Autodesk Inventor part; units mm, degrees
ref_plane "YZ Plane" through (0, 0, 0) normal (1, 0, 0) x (0, 1, 0)
ref_plane "XZ Plane" through (0, 0, 0) normal (0, 1, 0) x (-1, 0, 0)
ref_plane "XY Plane" through (0, 0, 0) normal (0, 0, 1) x (1, 0, 0)
sketch "Sketch1" plane through (0, 0, 0) normal (0, 0, 1) x (1, 0, 0)
  line L0 (52.5, 53) -> (52.5, -53)
  line L1 (-52.5, 53) -> (52.5, 53)
  line L2 (52.5, 53) -> (-52.5, 53)
  line L3 (-52.5, 53) -> (-52.5, -53)
  line L4 (-52.5, -53) -> (52.5, -53)
  line L5 (52.5, -53) -> (52.5, 53)
  line L6 (50.5, -51) -> (50.5, 51)
  line L7 (50.5, 51) -> (-50.5, 51)
  line L8 (50.5, 51) -> (-50.5, 51)
  line L9 (-50.5, 51) -> (-50.5, -51)
  line L10 (-50.5, -51) -> (50.5, -51)
  line L11 (50.5, -51) -> (50.5, 51)
  point P0 (0, 0)
extrude "Extrusion1" add sketch "Sketch1" along normal blind 10
sketch "Sketch2" plane through (0, 0, 0) normal (0, 0, -1) x (-1, 0, 0)
  circle A0 centre (-46, 46.5) radius 1.5
  line L0 (-50.5, 51) -> (-50.5, 42)
  line L1 (-41.5, 51) -> (-50.5, 51)
  line L2 (-41.5, 51) -> (-41.5, 42)
  line L3 (-41.5, 42) -> (-50.5, 42)
  circle A1 centre (-46, -46.5) radius 1.5
  line L4 (-41.5, -42) -> (-41.5, -51)
  line L5 (-50.5, -51) -> (-41.5, -51)
  line L6 (-50.5, -42) -> (-50.5, -51)
  line L7 (-50.5, -42) -> (-41.5, -42)
  circle A2 centre (46, -46.5) radius 1.5
  line L8 (50.5, -51) -> (50.5, -42)
  line L9 (41.5, -51) -> (50.5, -51)
  line L10 (41.5, -51) -> (41.5, -42)
  line L11 (41.5, -42) -> (50.5, -42)
  circle A3 centre (46, 46.5) radius 1.5
  line L12 (41.5, 42) -> (41.5, 51)
  line L13 (50.5, 51) -> (41.5, 51)
  line L14 (50.5, 42) -> (50.5, 51)
  line L15 (50.5, 42) -> (41.5, 42)
  point P0 (0, 0)
extrude "Extrusion2" add sketch "Sketch2" against normal blind 10
sketch "Sketch3" plane through (0, 0, 10) normal (0, 0, 1) x (1, 0, 0)
  line L0 (43.467, -7.68) -> (39.533, -7.68)
  line L1 (39.533, -7.68) -> (39.533, -6.68)
  line L2 (39.533, -6.68) -> (43.467, -6.68)
  line L3 (43.467, -6.68) -> (43.467, -7.68)
  line L4 (41.5, 42) -> (41.5, 51)
  line L5 (41.5, 51) -> (-41.5, 51)
  line L6 (-41.5, 51) -> (-41.5, 42)
  line L7 (-41.5, 42) -> (-50.5, 42)
  line L8 (-50.5, 42) -> (-50.5, -42)
  line L9 (-50.5, -42) -> (-41.5, -42)
  line L10 (-41.5, -42) -> (-41.5, -51)
  line L11 (-41.5, -51) -> (41.5, -51)
  line L12 (41.5, -51) -> (41.5, -42)
  line L13 (41.5, -42) -> (50.5, -42)
  line L14 (50.5, -42) -> (50.5, 42)
  line L15 (50.5, 42) -> (41.5, 42)
  line L16 (43.467, -7.68) -> (39.533, -7.68)
  line L17 (39.533, -7.68) -> (39.533, -6.68)
  line L18 (39.533, -6.68) -> (43.467, -6.68)
  line L19 (43.467, -6.68) -> (43.467, -7.68)
  line L20 (41.5, 42) -> (41.5, 51)
  line L21 (41.5, 51) -> (-41.5, 51)
  line L22 (-41.5, 51) -> (-41.5, 42)
  line L23 (-41.5, 42) -> (-50.5, 42)
  line L24 (-50.5, 42) -> (-50.5, -42)
  line L25 (-50.5, -42) -> (-41.5, -42)
  line L26 (-41.5, -42) -> (-41.5, -51)
  line L27 (-41.5, -51) -> (41.5, -51)
  line L28 (41.5, -51) -> (41.5, -42)
  line L29 (41.5, -42) -> (50.5, -42)
  line L30 (50.5, -42) -> (50.5, 42)
  line L31 (50.5, 42) -> (41.5, 42)
  circle A0 centre (44.2752, 10.8885) radius 1.8923
  circle A1 centre (-22.2674, 46.7091) radius 1.9651
  line L32 (38.467, -7.68) -> (34.533, -7.68)
  line L33 (34.533, -7.68) -> (34.533, -6.68)
  line L34 (34.533, -6.68) -> (38.467, -6.68)
  line L35 (38.467, -6.68) -> (38.467, -7.68)
  circle A2 centre (-36.634, 10.3057) radius 1.9118
  circle A3 centre (44.2752, 10.8885) radius 1.8923
  circle A4 centre (-22.2674, 46.7091) radius 1.9651
  line L36 (38.467, -7.68) -> (34.533, -7.68)
  line L37 (34.533, -7.68) -> (34.533, -6.68)
  line L38 (34.533, -6.68) -> (38.467, -6.68)
  line L39 (38.467, -6.68) -> (38.467, -7.68)
  circle A5 centre (-36.634, 10.3057) radius 1.9118
  point P0 (0, 0)
extrude "Extrusion3" add sketch "Sketch3" against normal blind 5 contours L0 L1 L2 L3 | L15 L14 L13 L12 L11 L10 L9 L8 L7 L6 L5 L4 | A0 | A1 | L32 L33 L34 L35 | A2
sketch "Sketch4" plane through (0, 0, 10) normal (0, 0, 1) x (1, 0, 0)
  circle A0 centre (46, 46.5) radius 1.5
  circle A1 centre (46, -46.5) radius 1.5
  circle A2 centre (-46, -46.5) radius 1.5
  circle A3 centre (-46, 46.5) radius 1.5
  circle A4 centre (46, 46.5) radius 4
  circle A5 centre (46, -46.5) radius 4
  circle A6 centre (-46, -46.5) radius 4
  circle A7 centre (-46, 46.5) radius 4
  point P0 (0, 0)
  dimension "d6" = 8
  dimension "d7" = 8
  dimension "d8" = 8
  dimension "d9" = 8
extrude "Extrusion4" cut sketch "Sketch4" against normal blind 8
sketch "Sketch5" plane through (0, 0, 10) normal (0, 0, 1) x (1, 0, 0)
  line L0 (-52.5, -53) -> (52.5, -53)
  line L1 (52.5, -53) -> (52.5, 53)
  line L2 (-52.5, -53) -> (52.5, -53)
  line L3 (52.5, -53) -> (52.5, 53)
  line L4 (52.5, 53) -> (-52.5, 53)
  line L5 (-52.5, 53) -> (-52.5, -53)
  line L6 (-52.5, 53) -> (-52.5, 0)
  circle A0 centre (0, 0) radius 10
  line L7 (-52.5, 0) -> (-42.5, 0)
  line L8 (-42.5, 0) -> (-42.5, 4)
  line L9 (-42.5, 4) -> (-33.5, 4)
  line L10 (-33.5, 4) -> (-33.5, -4)
  line L11 (-33.5, -4) -> (-42.5, -4)
  line L12 (-42.5, -4) -> (-42.5, 0)
  line L13 (-33.5, 0) -> (-10, 0)
  line L14 (-10, 0) -> (-21.75, 0)
  circle A1 centre (-21.75, 0) radius 7
  line L15 (0, 0) -> (21.75, 0)
  line L16 (42.5, 0) -> (42.5, -4)
  line L17 (42.5, -4) -> (33.5, -4)
  line L18 (33.5, -4) -> (33.5, 4)
  line L19 (33.5, 4) -> (42.5, 4)
  line L20 (42.5, 4) -> (42.5, 0)
  circle A2 centre (21.75, 0) radius 7
  point P0 (33.5, 0)
  dimension "d12" = 20
  dimension "d14" = 10
  dimension "d15" = 4
  dimension "d16" = 9
  dimension "d17" = 8
  dimension "d18" = 14
  dimension "d19" = 21.75
  dimension "d20" = 4
  dimension "d21" = 9
  dimension "d22" = 8
  dimension "d23" = 14
extrude "Extrusion5" cut sketch "Sketch5" against normal blind 4 contours A0
extrude "Extrusion6" cut sketch "Sketch5" against normal blind 2.2 contours A2 | A1 L13 | L13 A1
extrude "Extrusion7" cut sketch "Sketch5" against normal blind 1.5 contours L8 L9 L10 L11 L12 | L16 L17 L18 L19 L20
sketch "Sketch6" plane through (0, 0, 0) normal (0, 0, -1) x (-1, 0, 0)
  line L0 (-41.5, 42) -> (-41.5, 51)
  line L1 (-50.5, 42) -> (-41.5, 42)
  line L2 (-50.5, -42) -> (-50.5, 42)
  line L3 (-41.5, -42) -> (-50.5, -42)
  line L4 (-41.5, -51) -> (-41.5, -42)
  line L5 (41.5, -51) -> (-41.5, -51)
  line L6 (41.5, -42) -> (41.5, -51)
  line L7 (50.5, -42) -> (41.5, -42)
  line L8 (50.5, 42) -> (50.5, -42)
  line L9 (41.5, 42) -> (50.5, 42)
  line L10 (41.5, 51) -> (41.5, 42)
  line L11 (-41.5, 51) -> (41.5, 51)
  circle A0 centre (-46, 46.5) radius 1.5
  circle A1 centre (-46, -46.5) radius 1.5
  circle A2 centre (46, -46.5) radius 1.5
  circle A3 centre (46, 46.5) radius 1.5
  line L12 (-52.5, -53) -> (-52.5, 53)
  line L13 (52.5, -53) -> (-52.5, -53)
  line L14 (52.5, 53) -> (52.5, -53)
  line L15 (-52.5, 53) -> (52.5, 53)
  line L16 (-50.5, 42) -> (-50.5, -42)
  line L17 (-50.5, 42) -> (-41.5, 42)
  line L18 (-41.5, 42) -> (-41.5, 51)
  line L19 (41.5, 51) -> (-41.5, 51)
  line L20 (41.5, 51) -> (41.5, 42)
  line L21 (41.5, 42) -> (50.5, 42)
  line L22 (50.5, -42) -> (50.5, 42)
  line L23 (50.5, -42) -> (41.5, -42)
  line L24 (41.5, -42) -> (41.5, -51)
  line L25 (-41.5, -51) -> (41.5, -51)
  line L26 (-41.5, -51) -> (-41.5, -42)
  line L27 (-41.5, -42) -> (-50.5, -42)
  line L28 (41.5, -51) -> (50.5, -51)
  line L29 (50.5, -51) -> (50.5, -42)
  line L30 (-41.5, -51) -> (-50.5, -51)
  line L31 (-50.5, -51) -> (-50.5, -42)
  line L32 (-50.5, 42) -> (-50.5, 51)
  line L33 (-50.5, 51) -> (-41.5, 51)
  line L34 (50.5, 42) -> (50.5, 51)
  line L35 (50.5, 51) -> (41.5, 51)
  point P0 (0, 0)
extrude "Extrusion8" add sketch "Sketch6" along normal blind 0.5 contours L1 L32 L33 L0 | L35 L34 L9 L10 | L3 L4 L30 L31 | L29 L28 L6 L7
properties part number "parte superior"
Read the model definition and answer for the solid it produces. Units are mm, in the model's axes. A direction names the side the tool comes from. Coordinates: 2 decimals unless noted, no trailing zeros. Write each loop counter-clockwise with the first axis right and the second up, starting at its lowest first coordinate (ties: lowest second). Pieces come first, ordered by that corner, then holes. Notation, with made-up numbers: (54, 21) -> (94, 21) arc R6 cw to (94, 25) -> close; hole circle Ø5 at (5.25, 21). An arc over 180 degrees is marked (long way). Answer as a JSON object with one key per item and string values.
Q1. A tool of negligible diameter and unlimited length cuts with its end or side. For faces 1 (the flat face through (41.5, -46, 2)), 2 (the flat face through (47, 48, -0.5)), 3 (the flat face through (-22, 0, 7.8)), from which of +Z, -Z, +X, -X, +Y, -Y can it reach the whole face along a straight path? Write none if from no direction.
The answers:
{"face 1": "-Z", "face 2": "-Z, +X, -X, +Y, -Y", "face 3": "+Z"}
Q2. Flat-ended cylindrical pins translate along their axes: pin 1 Ø4 at (x, y) = (35.5, -18) entering from -Z; pin 2 Ø6.5 at (x, y) = (-38.5, 1.5) entering from +Z; pin 3 Ø12.5 at (x, y) = (-21.75, 0) entering from +Z; pin 4 Ø4 at (x, y) = (36, 0) entering from +Z. Find the tip coordinate at first contact, or state that the pin passes through.
The answers:
{"pin 1": "stops at z = 5", "pin 2": "stops at z = 10", "pin 3": "stops at z = 7.8", "pin 4": "stops at z = 8.5"}
Q3. The part is cut by section C-C on y = 46.5. Give the vertices of the cut face in (x, z).
The answers:
{"outline": "(-52.5, 0) -> (-50.5, 0) -> (-50.5, -0.5) -> (-47.5, -0.5) -> (-47.5, 2) -> (-50, 2) -> (-50, 10) -> (-52.5, 10) -> close; (-44.5, -0.5) -> (-41.5, -0.5) -> (-41.5, 5) -> (41.5, 5) -> (41.5, -0.5) -> (44.5, -0.5) -> (44.5, 2) -> (42, 2) -> (42, 10) -> (-42, 10) -> (-42, 2) -> (-44.5, 2) -> close; (47.5, -0.5) -> (50.5, -0.5) -> (50.5, 0) -> (52.5, 0) -> (52.5, 10) -> (50, 10) -> (50, 2) -> (47.5, 2) -> close"}
Q4. The part is cut by section B-B on x = 46. Give the vertices of the cut face in (y, z), then the cut area to 3 significant figures.
The answers:
{"outline": "(-53, 0) -> (-51, 0) -> (-51, -0.5) -> (-48, -0.5) -> (-48, 2) -> (-50.5, 2) -> (-50.5, 10) -> (-53, 10) -> close; (-45, -0.5) -> (-42, -0.5) -> (-42, 5) -> (42, 5) -> (42, -0.5) -> (45, -0.5) -> (45, 2) -> (42.5, 2) -> (42.5, 10) -> (-42.5, 10) -> (-42.5, 2) -> (-45, 2) -> close; (48, -0.5) -> (51, -0.5) -> (51, 0) -> (53, 0) -> (53, 10) -> (50.5, 10) -> (50.5, 2) -> (48, 2) -> close", "area": "506 mm2"}
Q5. The part is cut by section D-D on x = -21.75. Give the vertices of the cut face in (y, z).
The answers:
{"outline": "(-53, 0) -> (-51, 0) -> (-51, 5) -> (51, 5) -> (51, 0) -> (53, 0) -> (53, 10) -> (7, 10) -> (7, 7.8) -> (-7, 7.8) -> (-7, 10) -> (-53, 10) -> close"}
Q6. The part is cut by section A-A on z = 3.5. Give the vertices of the cut face in (x, y), then the cut area to 3 significant figures.
The answers:
{"outline": "(-52.5, -53) -> (52.5, -53) -> (52.5, 53) -> (-52.5, 53) -> close; hole (-50.5, -42) -> (-41.5, -42) -> (-41.5, -51) -> (41.5, -51) -> (41.5, -42) -> (50.5, -42) -> (50.5, 42) -> (41.5, 42) -> (41.5, 51) -> (-41.5, 51) -> (-41.5, 42) -> (-50.5, 42) -> close; hole circle Ø8 at (-46, -46.5); hole circle Ø8 at (-46, 46.5); hole circle Ø8 at (46, -46.5); hole circle Ø8 at (46, 46.5)", "area": "951 mm2"}
Q7. Consider line 1 (X direction, y = 46.5, z = 1.25); line 2 (X direction, y = 0, z = 9.45); line 3 (Y direction, x = 46, z = 0.8). Determine where each line is inside the solid, lowest interval first. Write a range as [from, to].
The answers:
{"line 1": "x = [-52.5, -47.5], [-44.5, -41.5], [41.5, 44.5], [47.5, 52.5]", "line 2": "x = [-52.5, -42.5], [-33.5, -28.75], [-14.75, -10], [10, 14.75], [28.75, 33.5], [42.5, 52.5]", "line 3": "y = [-53, -48], [-45, -42], [42, 45], [48, 53]"}
Q8. Determine the mould class of faces 4 (the cylindrical face through (-44.8, -45.6, 0.8)), 5 (the flat face through (52.5, 1, 5)), 6 (the flat face through (-1, -53, 5)) for opening direction X: pulls with the +X half, pulls with the -X half, needs draft (parallel to the pull), parting line crosses it, or undercut.
The answers:
{"face 4": "undercut", "face 5": "pulls with the +X half", "face 6": "needs draft"}
